For this review, take the finished solid that the model builds, in its own axes (mm). Face numbers are marked on the shaded views. A direction names the side the tool comes from. Coordinates: 2 decimals unless noted, no trailing zeros. Order: outer loops, then holes, each group sorted by start corner. A loop starts at its lowest first (then second) coordinate and runs counter-clockwise, first axis right, second up. Notation, with made-up numbers: (-11, 2) -> (-5, 2) arc R27 ccw to (-5, 21) -> close; hole circle Ø7 at (64, 51.25). An arc over 180 degrees is marked (long way). Answer as a JSON object with one key per item and string values. Group by question number.
1) Add section A-A, the plane z = 29. Write out the cut boundary in (x, y).
2) Add section D-D, the plane x = 49. Write out the cut boundary in (y, z).
3) For pin 1 (10 mm diameter, centred on x = -67, z = 21, fed in from -Y); pin 2 (11 mm diameter, centred on x = 83.5, z = 39.5, fed in from +Y); pin 3 (10.5 mm diameter, centred on x = 42.5, y = 2, fed in from +Z), all flat-tipped, find the tip position at first contact; note any pin that passes through.
4) Wall thickness on L1, parallel to X at y = -19, z = 21; L2, parallel to Y at x = 16, z = 12.5; L3, parallel to Z at x = -15, y = 2: over which ranges is each line inside the solid? List them lowest first.
5) Draft analysis for pull direction X (two halves, no side actions). For the marked faces 1, 2, 3 and 4, state which applies: +X half, -X half, draft (parallel to the pull), parting line (faces both ways), or undercut.
6) Machinability: for the marked faces 5, 6 and 7, which of the approach directions +Z, -Z, +X, -X, +Y, -Y give a long, thin tool a straight path to every point of the face, cutting with its end or side? Answer none if there is none.
7) Add section B-B, the plane y = -14. Write out the cut boundary in (x, z), then the cut area to 3 significant figures.
8) Add section C-C, the plane z = 12. Write out the cut boundary in (x, y).
from build123d import *

# Parameters (mm, degrees)
SKETCH2_W                      = 156
SKETCH2_H                      = 20
BASE_FLANGE1_DEPTH             = 10
EDGE_FLANGE1_STRIP_W           = 50
EDGE_FLANGE1_STRIP_H           = 10
EDGE_FLANGE1_STRIP_CUT_DEPTH   = 20
EDGE_FLANGE1_STRIP_2_W         = 50
EDGE_FLANGE1_STRIP_2_H         = 10
EDGE_FLANGE1_STRIP_CUT_2_DEPTH = 20
EDGE_FLANGE1_DEPTH             = 20
EDGE_FLANGE1_BEND_DEPTH        = 20
SKETCH15_W                     = 10
SKETCH15_H                     = 50
BOSS_EXTRUDE1_DEPTH            = 10
FILLET3_R                      = 5


# Sheet-metal steps are written as plain solids
with BuildPart() as part:
    # Sketch2 → Base-Flange1 (new body)
    with BuildSketch(Plane(origin=(0, 0, 0), x_dir=(1, 0, 0), z_dir=(0, 1, 0))):
        with Locations((0, -10)):
            Rectangle(SKETCH2_W, SKETCH2_H)
    extrude(amount=BASE_FLANGE1_DEPTH)

    # Edge-Flange1 strip (across the edge) → Edge-Flange1 strip cut (cut)
    with BuildSketch(Plane(origin=(-78, 0, 20), x_dir=(1, 0, 0), z_dir=(0, 0, -1))):
        with Locations((-20, -5)):
            Rectangle(EDGE_FLANGE1_STRIP_W, EDGE_FLANGE1_STRIP_H)
    extrude(amount=EDGE_FLANGE1_STRIP_CUT_DEPTH, mode=Mode.SUBTRACT)

    # Edge-Flange1 strip 2 (across the edge) → Edge-Flange1 strip cut 2 (cut)
    with BuildSketch(Plane(origin=(78, 0, 0), x_dir=(-1, 0, 0), z_dir=(0, 0, 1))):
        with Locations((-20, -5)):
            Rectangle(EDGE_FLANGE1_STRIP_2_W, EDGE_FLANGE1_STRIP_2_H)
    extrude(amount=EDGE_FLANGE1_STRIP_CUT_2_DEPTH, mode=Mode.SUBTRACT)

    # Edge-Flange1 section (across the edge) → Edge-Flange1 (add)
    with BuildSketch(Plane(origin=(-78, 0, 20), x_dir=(1, 0, 0), z_dir=(0, 0, -1))):
        with BuildLine():
            Line((-10, 5), (-10, 26))
            Line((-10, 26), (0, 26))
            Line((0, 26), (0, 5))
            ThreePointArc((0, 5), (1.464466094, 1.464466094), (5, 0))
            Line((5, 0), (5, -10))
            ThreePointArc((5, -10), (-5.606601718, -5.606601718), (-10, 5))
        make_face()
    extrude(amount=EDGE_FLANGE1_DEPTH)

    # Edge-Flange1 section 2 (across the edge) → Edge-Flange1 bend (add)
    with BuildSketch(Plane(origin=(78, 0, 0), x_dir=(-1, 0, 0), z_dir=(0, 0, 1))):
        with BuildLine():
            Line((-10, 5), (-10, 26))
            Line((-10, 26), (0, 26))
            Line((0, 26), (0, 5))
            ThreePointArc((0, 5), (1.464466094, 1.464466094), (5, 0))
            Line((5, 0), (5, -10))
            ThreePointArc((5, -10), (-5.606601718, -5.606601718), (-10, 5))
        make_face()
    extrude(amount=EDGE_FLANGE1_BEND_DEPTH)

    # Sketch15 → Boss-Extrude1 (add)
    with BuildSketch(Plane.XZ.offset(26)):
        with Locations((-83, 25)):
            Rectangle(SKETCH15_W, SKETCH15_H)
        with Locations((83, 25)):
            Rectangle(SKETCH15_W, SKETCH15_H)
    extrude(amount=-BOSS_EXTRUDE1_DEPTH)

    # Fillet3
    fillet3_edges = [part.edges().sort_by_distance(p)[0] for p in [
        (83, -16, 20),
        (-83, -16, 20),
    ]]
    fillet(fillet3_edges, radius=FILLET3_R)


solid = part.part
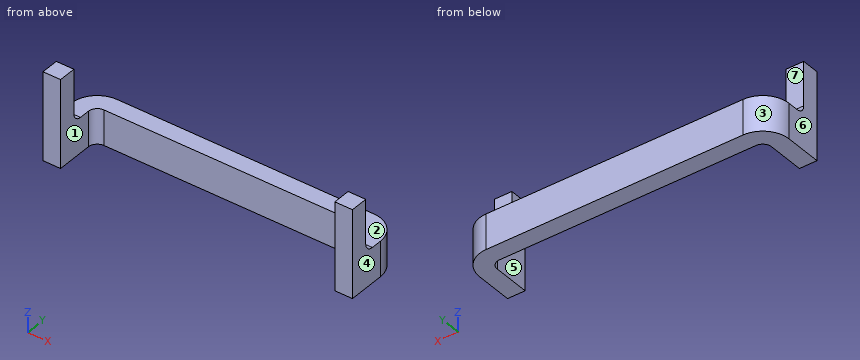
Output values:
{
 "1": {"outline": "(-88, -26) -> (-78, -26) -> (-78, -16) -> (-88, -16) -> close; (78, -26) -> (88, -26) -> (88, -16) -> (78, -16) -> close"},
 "2": {"outline": "(0, 0) -> (10, 0) -> (10, 20) -> (0, 20) -> close"},
 "3": {"pin 1": "stops at y = 0", "pin 2": "stops at y = -16", "pin 3": "stops at z = 20"},
 "4": {"L1": "x = -88 to -78, 78 to 88", "L2": "y = 0 to 10", "L3": "z = 0 to 20"},
 "5": {"face 1": "undercut", "face 2": "draft", "face 3": "-X half", "face 4": "+X half"},
 "6": {"face 5": "+Z, -Z, -Y", "face 6": "+Z, -Z, -X, +Y, -Y", "face 7": "+Z, +X, -X, +Y"},
 "7": {"outline": "(-88, 0) -> (-78, 0) -> (-78, 21) -> (-88, 21) -> close; (78, 0) -> (88, 0) -> (88, 21) -> (78, 21) -> close", "area": "420 mm²"},
 "8": {"outline": "(-88, -26) -> (-78, -26) -> (-78, -5) arc R5 cw to (-73, 0) -> (73, 0) arc R5 cw to (78, -5) -> (78, -26) -> (88, -26) -> (88, -5) arc R15 ccw to (73, 10) -> (-73, 10) arc R15 ccw to (-88, -5) -> close"}
}
